Autodesk Inventor part; units mm, degrees
ref_plane "YZ Plane" through (0, 0, 0) normal (1, 0, 0) x (0, 1, 0)
ref_plane "XZ Plane" through (0, 0, 0) normal (0, 1, 0) x (-1, 0, 0)
ref_plane "XY Plane" through (0, 0, 0) normal (0, 0, 1) x (1, 0, 0)
sketch "Sketch1" plane through (0, 0, 0) normal (0, 1, 0) x (-1, 0, 0)
  line L0 (-5.5, 3.1754) -> (0, 6.3509)
  line L1 (0, 6.3509) -> (5.5, 3.1754)
  line L2 (5.5, 3.1754) -> (5.5, -3.1754)
  line L3 (5.5, -3.1754) -> (0, -6.3509)
  line L4 (0, -6.3509) -> (-5.5, -3.1754)
  line L5 (-5.5, -3.1754) -> (-5.5, 3.1754)
  point P0 (0, 0)
  point P1 (0, 0)
  dimension "d0" = 11
extrude "Extrusion1" add sketch "Sketch1" along normal blind 2
sketch "Sketch2" plane through (0, 2, 0) normal (0, 1, 0) x (1, 0, 0)
  circle A0 centre (0, 0) radius 4.3
  dimension "d3" = 8.6
extrude "Extrusion2" add sketch "Sketch2" along normal blind 2
sketch "Sketch3" plane through (0, 4, 0) normal (0, 1, 0) x (1, 0, 0)
  circle A0 centre (0, 0) radius 4
  circle A1 centre (0, 0) radius 4.3
  dimension "d6" = 8
hole "Hole1" at (0, 4, 0) direction (0, -1, 0) diameter 6.647 end through all
properties part number "Pot Adaptor"
Verification items for the finished model (mm, model axes). A direction names the side the tool comes from. Round coordinates to 2 decimals unless told otherwise and drop trailing zeros. Order: outer loops, then holes, each group sorted by start corner. A loop starts at its lowest first (then second) coordinate and runs counter-clockwise, first axis right, second up. Notation, with made-up numbers: (26.25, 20) - (43.25, 20) arc R25 ccw to (43.25, 33) - close; hole circle Ø2 at (-17.5, -39.5). An arc over 180 degrees is marked (long way). Use CSV: the item, a comma, the result in double quotes. Start each with the question number.
1) Section check A-A, the plane z = 0. Record the cut outline in (x, y).
2) Section check B-B, the plane y = 1.8. Record the cut outline in (x, z).
3) Go/stop test with flat-tipped pins: P1, Ø5.5, axis at x = 0.5, z = 3, coming from the +Y side; P2, Ø1, axis at y = 3, z = -3, coming from the -X side. Record where each tip stops, or that it passes through.
4) Section check D-D, the plane y = 3.45. Record the cut outline in (x, z).
5) Access from +Z, -Z, +X, -X, +Y, -Y to the whole of each face (thin tool, end or side, straight path). Record for faces 5 (the cylindrical face through (-4.296, 2.986, 0.189)), 6 (the flat face through (2, 4, 3)).
6) Mould release check, pull along X, two halves, no side actions. Record for faces 1 (the flat face through (2.712, 0.986, -4.785)), 2 (the flat face through (-2.712, 0.986, 4.785)), 3 (the cylindrical face through (1.27, 1.97, 3.07)), 4 (the flat face through (4, 2, -2)): +X half, -X half, draft (parallel to the pull), parting line (faces both ways), or undercut.
7) Thickness scan on L1, parallel to X at y = 2.9, z = 0; L2, parallel to X at y = 1.95, z = 0. Record the ranges inside material, lowest first.
8) Section check C-C, the plane z = 2. Record the cut outline in (x, y).
Answers:
1,outline,"(-5.5, 0) - (-3.32, 0) - (-3.32, 4) - (-4.3, 4) - (-4.3, 2) - (-5.5, 2) - close; (3.32, 0) - (5.5, 0) - (5.5, 2) - (4.3, 2) - (4.3, 4) - (3.32, 4) - close"
2,outline,"(-5.5, -3.18) - (0, -6.35) - (5.5, -3.18) - (5.5, 3.18) - (0, 6.35) - (-5.5, 3.18) - close; hole circle Ø6.65 at (0, 0)"
3,P1,"stops at y = 4"
3,P2,"stops at x = -3.5"
4,outline,"circle Ø8.6 at (0, 0); hole circle Ø6.65 at (0, 0)"
5,face 5,"+Y"
5,face 6,"+Z, -Z, +X, -X, +Y"
6,face 1,"+X half"
6,face 2,"-X half"
6,face 3,"undercut"
6,face 4,"draft"
7,L1,"x = -4.3 to -3.32, 3.32 to 4.3"
7,L2,"x = -5.5 to -3.32, 3.32 to 5.5"
8,outline,"(-5.5, 0) - (-2.65, 0) - (-2.65, 4) - (-3.81, 4) - (-3.81, 2) - (-5.5, 2) - close; (2.65, 0) - (5.5, 0) - (5.5, 2) - (3.81, 2) - (3.81, 4) - (2.65, 4) - close"
